Source: three-view drawing plus pictorial views. Frame: mm from the lowest corner of the part. A direction names the side the tool comes from. Give positions to 0.01 mm unless a question says otherwise; leave off trailing zeros. Order: outer loops, then holes, each group sorted by start corner. A loop starts at its lowest first (then second) coordinate and runs counter-clockwise, first axis right, second up. Notation, with made-up numbers: M 74.25,-2 L 127.25,-2 A24 cw 127.25,37 Z; hole C -11,-4 d11. An arc over 180 degrees is marked long. One line per item, written item: value. Start each with the question number.
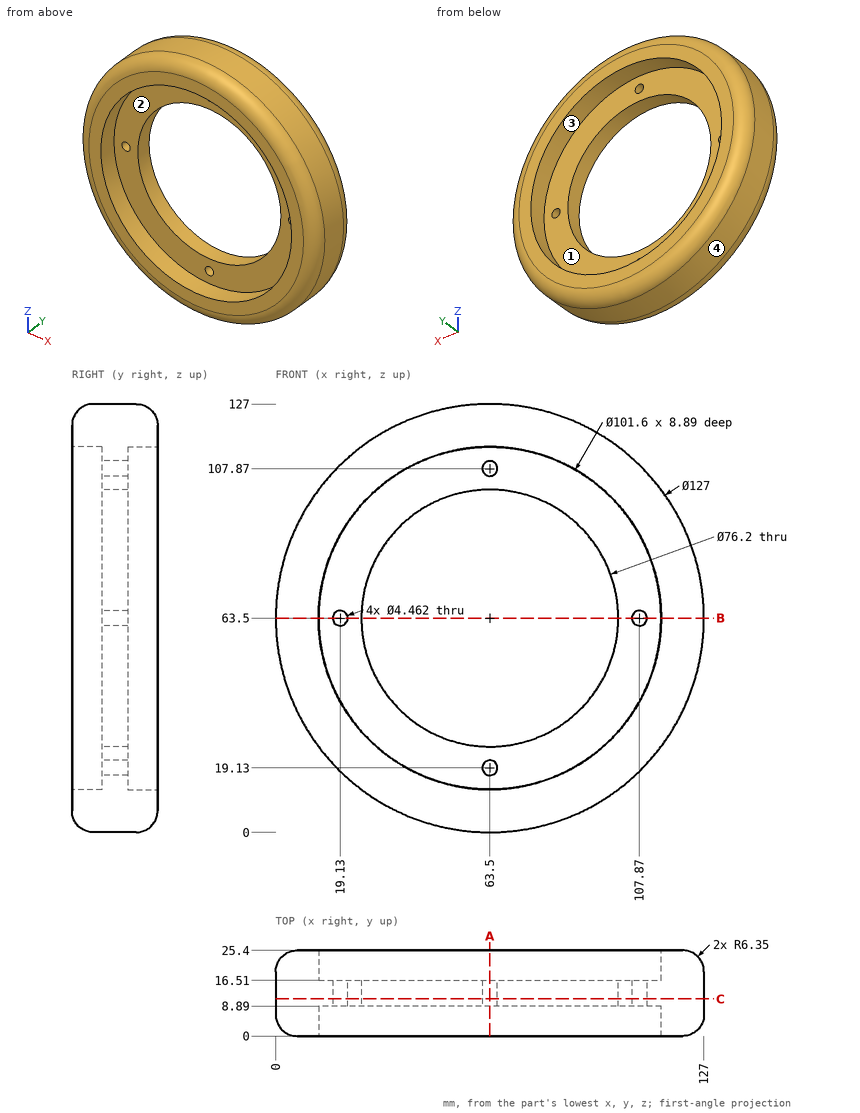
Q1. Mould query, pull axis Z, two halves, no side actions, for the marked faces 3 and 4. Classes: +Z half, -Z half, draft (parallel to the pull), parting line (faces both ways), or undercut.
Q2. Section query B-B on z = 63.5. Return loops of the section in (x, y), and give its area (3 significant figures).
Q3. Contact query for flat-ended pins moving along their axis: pin 1 (2 mm diameter, centred on x = 89, y = 22.5, fed in from -Z) (1 decimal); pin 2 (8 mm diameter, centred on x = 43.5, y = 21.5, fed in from +Z) (1 decimal); pin 3 (12 mm diameter, centred on y = 9, z = 75, fed in from -X). Output: stop coordinate, or through.
Q4. Set-up query: the marked faces 1 and 2. Return all of +Z, -Z, +X, -X, +Y, -Y with unobstructed straight access to the full face (end or side cutting, diameter ignored); none if empty.
Q5. Ray query, line 1 along Z through (x, y) = (63.5, 14.25); line 2 along Y through (x, z) = (75, 104); line 3 along X through (y, z) = (18.25, 87). Return the intervals inside material, ascending. Write a range as [from, to].
Q6. Section query A-A on x = 63.5. Return loops of the section in (y, z).
Q7. Section query C-C on y = 11. Return loops of the section in (x, z).
Results below:
1. face 3: undercut
1. face 4: parting line
2. outline: M 0,6.35 A6.35 ccw 6.35,0 L 12.7,0 L 12.7,8.89 L 16.9,8.89 L 16.9,16.51 L 12.7,16.51 L 12.7,25.4 L 6.35,25.4 A6.35 ccw 0,19.05 Z; M 21.36,8.89 L 25.4,8.89 L 25.4,16.51 L 21.36,16.51 Z; M 101.6,8.89 L 105.64,8.89 L 105.64,16.51 L 101.6,16.51 Z; M 110.1,8.89 L 114.3,8.89 L 114.3,0 L 120.65,0 A6.35 ccw 127,6.35 L 127,19.05 A6.35 ccw 120.65,25.4 L 114.3,25.4 L 114.3,16.51 L 110.1,16.51 Z
2. area: 736 mm2
3. pin 1: z = 5.7
3. pin 2: z = 124.8
3. pin 3: x = 0.24
4. face 1: +Y
4. face 2: -Y
5. line 1: [0, 16.9], [21.36, 25.4], [101.6, 105.64], [110.1, 127]
5. line 2: [8.89, 16.51]
5. line 3: [4.51, 18.46], [108.54, 122.49]
6. outline: M 0,6.35 A6.35 ccw 6.35,0 L 19.05,0 A6.35 ccw 25.4,6.35 L 25.4,12.7 L 16.51,12.7 L 16.51,16.9 L 8.89,16.9 L 8.89,12.7 L 0,12.7 Z; M 0,114.3 L 8.89,114.3 L 8.89,110.1 L 16.51,110.1 L 16.51,114.3 L 25.4,114.3 L 25.4,120.65 A6.35 ccw 19.05,127 L 6.35,127 A6.35 ccw 0,120.65 Z; M 8.89,21.36 L 16.51,21.36 L 16.51,25.4 L 8.89,25.4 Z; M 8.89,101.6 L 16.51,101.6 L 16.51,105.64 L 8.89,105.64 Z
7. outline: C 63.5,63.5 d127; hole C 19.13,63.5 d4.46; hole C 63.5,63.5 d76.2; hole C 63.5,19.13 d4.46; hole C 63.5,107.87 d4.46; hole C 107.87,63.5 d4.46
